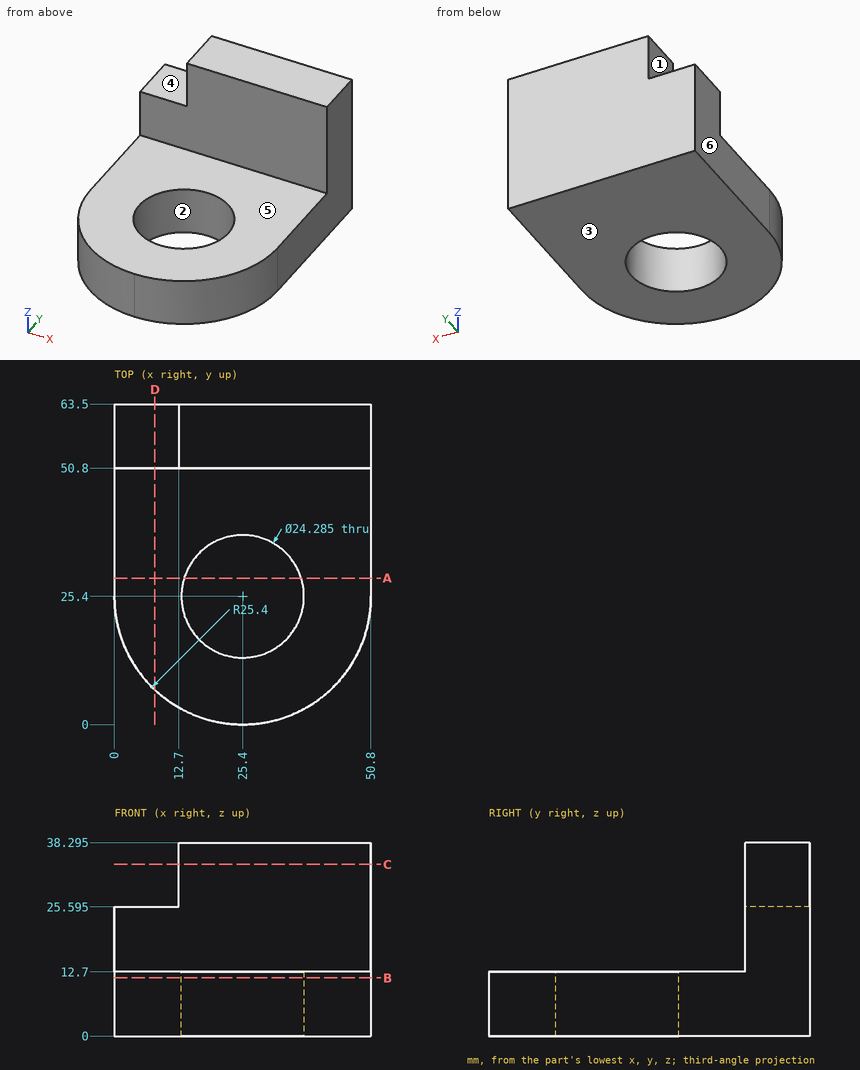
Job drawing, mm, ordinate dimensions from the low corner. One solid piece. A direction names the side the tool comes from. Give positions to 0.01 mm unless a question says otherwise; leave off trailing zeros. Loops run counter-clockwise (first coordinate to the right, second up) from the corner with the lowest first, then second, coordinate; pieces in that order, holes last. Notation, with made-up numbers: (47.5, -17) -> (84.5, -17) arc R7 ccw to (84.5, -7) -> close; hole circle Ø3 at (10, 46). An arc over 180 degrees is marked (long way). Use a Markdown table: item, result. Add a question column.
(1) Mould opens along X. For the marked faces 1, 2 and 3 say: +X half, -X half, draft (parallel to the pull), parting line (faces both ways), or undercut.
(2) Wall check: line 1 along X through (y, z) = (25, 5) (1 decimal); line 2 along Y through (x, z) = (42.5, 34.5); line 3 along Y through (x, z) = (25, 8). Give the ranges that are in metal, low to high.
(3) Drop flat-ended pins along their axis: pin 1 Ø8 at (x, y) = (9, 43) entering from +Z; pin 2 Ø6 at (x, y) = (13, 30) entering from -Z; pin 3 Ø8 at (y, z) = (11.5, 5.5) entering from +X; pin 4 Ø4 at (y, z) = (60, 31) entering from -X. Give the stop position or say it passes through.
(4) Slice it at A-A on y = 29. List the corners of the cut face in (x, z), and give its area (3 significant figures).
(5) Slice it at D-D on x = 8. List the corners of the cut face in (y, z) (1 decimal), and give its area (3 significant figures).
(6) Slice it at C-C on z = 34. List the corners of the cut face in (x, y).
(7) Slice it at B-B on z = 11.5. List the corners of the cut face in (x, y) (1 decimal).
(8) Tool access for the marked faces 4, 5 and 6: list every direction of +Z, -Z, +X, -X, +Y, -Y with a clear straight run to the whole face (end or side of a thin tool).
Filled sheet:
| question | item | result |
|---|---|---|
| 1 | face 1 | -X half |
| 1 | face 2 | undercut |
| 1 | face 3 | draft |
| 2 | line 1 | 0 to 13.3, 37.5 to 50.8 |
| 2 | line 2 | 50.8 to 63.5 |
| 2 | line 3 | 0 to 13.26, 37.54 to 63.5 |
| 3 | pin 1 | z = 12.7 |
| 3 | pin 2 | z = 0 |
| 3 | pin 3 | x = 48.79 |
| 3 | pin 4 | x = 12.7 |
| 4 | outline | (0, 0) -> (13.8, 0) -> (13.8, 12.7) -> (0, 12.7) -> close; (37, 0) -> (50.8, 0) -> (50.8, 12.7) -> (37, 12.7) -> close |
| 4 | area | 351 mm2 |
| 5 | outline | (6.9, 0) -> (63.5, 0) -> (63.5, 25.6) -> (50.8, 25.6) -> (50.8, 12.7) -> (6.9, 12.7) -> close |
| 5 | area | 883 mm2 |
| 6 | outline | (12.7, 50.8) -> (50.8, 50.8) -> (50.8, 63.5) -> (12.7, 63.5) -> close |
| 7 | outline | (0, 25.4) arc R25.4 ccw to (25.4, 0) arc R25.4 ccw to (50.8, 25.4) -> (50.8, 63.5) -> (0, 63.5) -> close; hole circle Ø24.3 at (25.4, 25.4) |
| 8 | face 4 | +Z, -X, +Y, -Y |
| 8 | face 5 | +Z, +X, -X, -Y |
| 8 | face 6 | +Z, -Z, -X, +Y, -Y |
